Part model, mm, in its own coordinate system. A direction names the side the tool comes from. Coordinates: 2 decimals unless noted, no trailing zeros. Loops run counter-clockwise (first coordinate to the right, second up) from the corner with the lowest first, then second, coordinate; pieces in that order, holes last. Notation, with made-up numbers: (64.5, 64) - (76.5, 64) arc R21 ccw to (76.5, 93) - close; hole circle Ø9 at (48, 89). An arc over 180 degrees is marked (long way). Use a Markdown table: item, result. Add a question column.
1. 3-axis set-ups, long thin cutter, end or side, ignore diameter. For faces 4 (the flat face through (12.4, 16.65, 17.09)), 5 (the flat face through (-12.394, 16.627, 17.091)), 6 (the flat face through (-0.253, 20.736, 17.091)): which of +Z, -Z, +X, -X, +Y, -Y reach the whole face in a straight line?
2. Band-saw the part on D-D, the plane y = 23.5. Give the cut face in (x, z), plus the area to 3 significant figures.
3. Band-saw the part on A-A, the plane y = 0. Give the cut face in (x, z), plus the area to 3 significant figures.
4. Drop flat-ended pins along their axis: pin 1 (1.5 mm diameter, centred on x = -4.5, y = 18, fed in from -Z); pin 2 (8 mm diameter, centred on y = -1.5, z = 5.5, fed in from -X); pin 3 (1 mm diameter, centred on y = -7, z = 11.5, fed in from +X); pin 4 (3 mm diameter, centred on y = 18, z = 6.5, fed in from +X). Give the stop position or say it passes through.
5. Wall check: probe 1 along Y at (x, z) = (0, 10); probe 2 along Z at (x, y) = (25, -3.5); probe 3 along X at (y, z) = (17, 22.5). Give the ranges that are in metal, low to high. Write a range as [from, to].
6. Pull direction Z, two halves, no side cores. Call faces 1 (the flat face through (6, 0, 0)), 2 (the flat face through (6, 0, 35)), 3 (the flat face through (0.253, -20.736, 17.091)): pulls with the +Z half, pulls with the -Z half, needs draft (parallel to the pull), parting line crosses it, or undercut.
7. Band-saw the part on C-C, the plane x = -3.5. Give the cut face in (y, z).
from build123d import *

# Parameters (mm, degrees)
SKETCH_1_R               = 20
EXTRUDE_1_DEPTH          = 35
SKETCH_3_R               = 30
EXTRUDE_2_DEPTH          = 1
EXTRUDE_START            = -1
SKETCH_4_R               = 30
EXTRUDE_3_DEPTH          = 1
CUT_EXTRUDE_2_DEPTH      = 56
CUT_EXTRUDE_2_DEPTH_BACK = 56
SKETCH_5_W               = 1
SKETCH_5_H               = 13
EXTRUDE_4_DEPTH          = 21.5
CUT_EXTRUDE_3_REACH      = 50.5
PATTERN_CIRCULAR_2_COUNT = 10
CUT_EXTRUDE_5_DEPTH      = 56
CUT_EXTRUDE_5_DEPTH_BACK = 56
SKETCH_9_R               = 5
EXTRUDE_5_DEPTH          = 35
SKETCH_10_R              = 2
CUT_EXTRUDE_6_DEPTH      = 56


with BuildPart() as part:
    # Sketch 1 → Extrude 1 (new body)
    with BuildSketch(Plane.XY):
        Circle(SKETCH_1_R)
    extrude(amount=EXTRUDE_1_DEPTH)

    # Sketch 3 → Extrude 2 (add)
    with BuildSketch(Plane.XY.offset(35)):
        Circle(SKETCH_3_R)
    extrude(amount=-EXTRUDE_2_DEPTH)

    # Sketch 4 → Extrude 3 (add)
    with BuildSketch(Plane(origin=(0, 0, 0), x_dir=(-1, 0, 0), z_dir=(0, 0, -1)).offset(EXTRUDE_START)):
        with Locations(Location((0, 0, 0), (0, 0, 180))):
            Circle(SKETCH_4_R)
    extrude(amount=EXTRUDE_3_DEPTH)

    # Sketch 2 → Cut-Extrude 2 (cut, two sides: drawn at the far end of the back side and taken through both)
    with BuildSketch(Plane.XY.offset(35).offset(-CUT_EXTRUDE_2_DEPTH_BACK)):
        with BuildLine():
            Line((-1.944865034, 1.8), (1.944865034, 1.8))
            ThreePointArc((1.944865034, 1.8), (2.65, 0), (1.944865034, -1.8))
            Line((1.944865034, -1.8), (-1.944865034, -1.8))
            ThreePointArc((-1.944865034, -1.8), (-2.65, 0), (-1.944865034, 1.8))
        make_face()
    extrude(amount=CUT_EXTRUDE_2_DEPTH + CUT_EXTRUDE_2_DEPTH_BACK, mode=Mode.SUBTRACT)

    # Sketch 5 → Extrude 4 (add)
    with BuildSketch(Plane(origin=(0, 0, 0), x_dir=(1, 0, 0), z_dir=(0, 1, 0))):
        with Locations((0, -17)):
            Rectangle(SKETCH_5_W, SKETCH_5_H)
    extrude_4 = extrude(amount=EXTRUDE_4_DEPTH)

    # Sketch 6 → Cut-Extrude 3 (cut, up to next)
    with BuildSketch(Plane.XY.offset(23.5), mode=Mode.PRIVATE) as cut_extrude_3_sk1:
        Polygon((-0.5, 19.993749023), (0, 21.5), (-0.5, 21.5), align=None)
    cut_extrude_3_tool1 = extrude(cut_extrude_3_sk1.sketch, amount=-CUT_EXTRUDE_3_REACH, mode=Mode.PRIVATE) & part.part
    # Sketch 6 → Cut-Extrude 3 (cut, up to next)
    with BuildSketch(Plane.XY.offset(23.5), mode=Mode.PRIVATE) as cut_extrude_3_sk2:
        Polygon((0.5, 21.5), (0, 21.5), (0.5, 19.993749023), align=None)
    cut_extrude_3_tool2 = extrude(cut_extrude_3_sk2.sketch, amount=-CUT_EXTRUDE_3_REACH, mode=Mode.PRIVATE) & part.part
    cut_extrude_3_1 = cut_extrude_3_tool1.solids().sort_by_distance((-0.333333, 20.997916, 23.5))[0]
    add(cut_extrude_3_1, mode=Mode.SUBTRACT)
    cut_extrude_3_2 = cut_extrude_3_tool2.solids().sort_by_distance((0.333333, 20.997916, 23.5))[0]
    add(cut_extrude_3_2, mode=Mode.SUBTRACT)
    cut_extrude_3 = cut_extrude_3_1 + cut_extrude_3_2  # Cut-Extrude 3 as one shape, for the pattern or mirror that repeats it

    # Pattern Circular 2: Extrude 4, Cut-Extrude 3 ×10 about axis
    pattern_circular_2_axis = Axis((0, 0, 0), (0, 0, 1))
    add([extrude_4.rotate(pattern_circular_2_axis, i * 360 / PATTERN_CIRCULAR_2_COUNT) for i in range(1, PATTERN_CIRCULAR_2_COUNT)])
    add([cut_extrude_3.rotate(pattern_circular_2_axis, i * 360 / PATTERN_CIRCULAR_2_COUNT) for i in range(1, PATTERN_CIRCULAR_2_COUNT)], mode=Mode.SUBTRACT)

    # Sketch 8 → Cut-Extrude 5 (cut, two sides: drawn at the far end of the back side and taken through both)
    with BuildSketch(Plane.XY.offset(35).offset(-CUT_EXTRUDE_5_DEPTH_BACK)):
        with BuildLine():
            ThreePointArc((-1.944865034, -1.8), (-2.65, 0), (-1.944865034, 1.8))
            Line((-1.944865034, 1.8), (1.944865034, 1.8))
            ThreePointArc((1.944865034, 1.8), (2.65, 0), (1.944865034, -1.8))
            Line((1.944865034, -1.8), (-1.944865034, -1.8))
        make_face()
    extrude(amount=CUT_EXTRUDE_5_DEPTH + CUT_EXTRUDE_5_DEPTH_BACK, mode=Mode.SUBTRACT)

    # Sketch 9 → Extrude 5 (add, through all)
    with BuildSketch(Plane.XY.offset(35)):
        Circle(SKETCH_9_R)
    extrude(amount=-EXTRUDE_5_DEPTH)

    # Sketch 10 → Cut-Extrude 6 (cut, through all)
    with BuildSketch(Plane.XY.offset(35)):
        Circle(SKETCH_10_R)
    extrude(amount=-CUT_EXTRUDE_6_DEPTH, mode=Mode.SUBTRACT)


solid = part.part
Geometry check:
| question | item | result |
|---|---|---|
| 1 | face 4 | +X |
| 1 | face 5 | -X |
| 1 | face 6 | -X, +Y |
| 2 | outline | (-18.65, 0) - (18.65, 0) - (18.65, 1) - (-18.65, 1) - close; (-18.65, 34) - (18.65, 34) - (18.65, 35) - (-18.65, 35) - close |
| 2 | area | 74.6 mm^2 |
| 3 | outline | (-30, 0) - (-2, 0) - (-2, 35) - (-30, 35) - (-30, 34) - (-20, 34) - (-20, 1) - (-30, 1) - close; (2, 0) - (30, 0) - (30, 1) - (20, 1) - (20, 34) - (30, 34) - (30, 35) - (2, 35) - close |
| 3 | area | 1,300 mm^2 |
| 4 | pin 1 | stops at z = 0 |
| 4 | pin 2 | stops at x = -20 |
| 4 | pin 3 | stops at x = 20.45 |
| 4 | pin 4 | stops at x = 11.3 |
| 5 | probe 1 | y = [-20, -2], [2, 20] |
| 5 | probe 2 | z = [0, 1], [34, 35] |
| 5 | probe 3 | x = [-12.51, -12.09], [-10.54, 10.54], [12.09, 12.51] |
| 6 | face 1 | pulls with the -Z half |
| 6 | face 2 | pulls with the +Z half |
| 6 | face 3 | undercut |
| 7 | outline | (-29.8, 0) - (29.8, 0) - (29.8, 1) - (19.69, 1) - (19.69, 34) - (29.8, 34) - (29.8, 35) - (-29.8, 35) - (-29.8, 34) - (-19.69, 34) - (-19.69, 1) - (-29.8, 1) - close |
